```python
from build123d import *

# Parameters (mm, degrees)
SKETCH1_W           = 90
SKETCH1_H           = 35
SKETCH1_R           = 5.5
SKETCH1_R_2         = 1.5
SKETCH1_R_3         = 11
BOSS_EXTRUDE1_DEPTH = 6
SKETCH2_W           = 90
SKETCH2_H           = 3
BOSS_EXTRUDE2_DEPTH = 20
SKETCH4_R           = 2.5
CUT_EXTRUDE1_DEPTH  = 10
SKETCH5_R           = 2.7
CUT_EXTRUDE2_DEPTH  = 10


with BuildPart() as part:
    # Sketch1 → Boss-Extrude1 (new body)
    with BuildSketch(Plane.XY):
        Rectangle(SKETCH1_W, SKETCH1_H)
        with Locations((-30, 0)):
            Circle(SKETCH1_R, mode=Mode.SUBTRACT)
        with Locations((-38, 0)):
            Circle(SKETCH1_R_2, mode=Mode.SUBTRACT)
        with Locations((-22, 0)):
            Circle(SKETCH1_R_2, mode=Mode.SUBTRACT)
        with Locations((29.999666666, 0.2)):
            Circle(SKETCH1_R_3, mode=Mode.SUBTRACT)
    extrude(amount=BOSS_EXTRUDE1_DEPTH)

    # Sketch2 → Boss-Extrude2 (add)
    with BuildSketch(Plane.XY.offset(6)):
        with Locations((0, -16)):
            Rectangle(SKETCH2_W, SKETCH2_H)
    extrude(amount=-BOSS_EXTRUDE2_DEPTH)

    # Sketch4 → Cut-Extrude1 (cut)
    with BuildSketch(Plane.XY.offset(6)):
        with Locations((15, -7.5)):
            Circle(SKETCH4_R)
        with Locations(Location((-15, -7.5, 0), (0, 0, 180))):
            Circle(SKETCH4_R)
        with BuildLine():
            Line((2.5, 9.778989608), (2.5, 0.141519694))
            ThreePointArc((2.5, 0.141519694), (0, -2.358480306), (-2.5, 0.141519694))
            Line((-2.5, 0.141519694), (-2.5, 9.778989608))
            ThreePointArc((-2.5, 9.778989608), (0, 12.278989608), (2.5, 9.778989608))
        make_face()
    extrude(amount=-CUT_EXTRUDE1_DEPTH, mode=Mode.SUBTRACT)

    # Sketch5 → Cut-Extrude2 (cut)
    with BuildSketch(Plane(origin=(0, -14.5, 0), x_dir=(1, 0, 0), z_dir=(0, 1, 0))):
        with Locations(Location((30, 6.5, 0), (0, 0, 270))):
            Circle(SKETCH5_R)
        with Locations(Location((-30, 6.5, 0), (0, 0, 270))):
            Circle(SKETCH5_R)
    extrude(amount=-CUT_EXTRUDE2_DEPTH, mode=Mode.SUBTRACT)


solid = part.part
```
The model under review builds one solid part; all positions refer to its coordinate system, in mm. A direction names the side the tool comes from. Coordinates: 2 decimals unless noted, no trailing zeros. Write each loop counter-clockwise with the first axis right and the second up, starting at its lowest first coordinate (ties: lowest second). Pieces come first, ordered by that corner, then holes. Notation, with made-up numbers: (57, 33.5) - (93, 33.5) arc R25 ccw to (93, 71.5) - close; hole circle Ø3 at (-1.75, -7.5). An arc over 180 degrees is marked (long way). Answer in a Markdown table with one row per item. Add a question column.
Q1. Draft analysis for pull direction Y (two halves, no side actions). For faces 1 (the face through (-23.5, 0.07, 2.96)), 2 (the face through (-1, -14.5, -7)), 3 (the face through (-11, 2, 0)), 4 (the face through (0.055, -2.358, 3.042)), state which applies: +Y half, -Y half, draft (parallel to the pull), parting line (faces both ways), or undercut.
Q2. For faces 5 (the face through (32.277, -15.979, -5.048)), 6 (the face through (-2.5, 5, 3)), list the 3-axis set-ups (+Z, -Z, +X, -X, +Y, -Y) from which the entire face can be reached by the end or side of a thin tool; tool diameter is ignored.
Q3. Consider section D-D on y = 3.5. Give the boundary of the cut face in (x, z), then the cut area to 3 significant figures.
Q4. Consider section C-C on x = 15. Give the boundary of the cut face in (y, z), then the cut area to 3 significant figures.
Q5. Consider section B-B on z = -6.5. Give the boundary of the cut face in (x, y).
Q6. Consider section A-A on x = -30. Give the boundary of the cut face in (y, z), then the cut area to 3 significant figures.
Q7. To check wall thickness, follow line 1 along X through (y, z) = (-15.8, -6.5); line 2 along Y through (x, z) = (15, 2.6); line 3 along X through (y, z) = (3, 4). State the ranges of each line that lie inside material, in increasing order. Write a range as from..to.
Q8. Clearance check with flat-ended pins moving along their axes: pin 1 (1.8 mm diameter, centred on x = -22, y = 0, fed in from -Z); pin 2 (11 mm diameter, centred on x = 17, z = -8, fed in from +Y); pin 3 (1 mm diameter, centred on x = 22, y = -9.5, fed in from -Z). State where each tip first meets the part, or that it passes through.
Answers below:
| question | item | result |
|---|---|---|
| 1 | face 1 | undercut |
| 1 | face 2 | +Y half |
| 1 | face 3 | draft |
| 1 | face 4 | undercut |
| 2 | face 5 | +Y, -Y |
| 2 | face 6 | +Z, -Z |
| 3 | outline | (-45, 0) - (-34.24, 0) - (-34.24, 6) - (-45, 6) - close; (-25.76, 0) - (-2.5, 0) - (-2.5, 6) - (-25.76, 6) - close; (2.5, 0) - (19.51, 0) - (19.51, 6) - (2.5, 6) - close; (40.49, 0) - (45, 0) - (45, 6) - (40.49, 6) - close |
| 3 | area | 333 mm² |
| 4 | outline | (-17.5, -14) - (-14.5, -14) - (-14.5, 0) - (-10, 0) - (-10, 6) - (-17.5, 6) - close; (-5, 0) - (17.5, 0) - (17.5, 6) - (-5, 6) - close |
| 4 | area | 222 mm² |
| 5 | outline | (-45, -17.5) - (-32.7, -17.5) - (-32.7, -14.5) - (-45, -14.5) - close; (-27.3, -17.5) - (27.3, -17.5) - (27.3, -14.5) - (-27.3, -14.5) - close; (32.7, -17.5) - (45, -17.5) - (45, -14.5) - (32.7, -14.5) - close |
| 6 | outline | (-17.5, -14) - (-14.5, -14) - (-14.5, -9.2) - (-17.5, -9.2) - close; (-17.5, -3.8) - (-14.5, -3.8) - (-14.5, 0) - (-5.5, 0) - (-5.5, 6) - (-17.5, 6) - close; (5.5, 0) - (17.5, 0) - (17.5, 6) - (5.5, 6) - close |
| 6 | area | 170 mm² |
| 7 | line 1 | -45..-32.7, -27.3..27.3, 32.7..45 |
| 7 | line 2 | -17.5..-10, -5..17.5 |
| 7 | line 3 | -45..-34.61, -25.39..-2.5, 2.5..19.36, 40.64..45 |
| 8 | pin 1 | through |
| 8 | pin 2 | y = -14.5 |
| 8 | pin 3 | z = 0 |
